```python
from build123d import *

# Parameters (mm, degrees)
CROQUIS1_W              = 21
CROQUIS1_H              = 20
SALIENTE_EXTRUIR1_DEPTH = 5
CROQUIS2_R              = 1.35
CORTAR_EXTRUIR1_DEPTH   = 6
CROQUIS3_R              = 2.5
CORTAR_EXTRUIR2_DEPTH   = 2
CROQUIS4_R              = 2.1
CORTAR_EXTRUIR3_DEPTH   = 6
CROQUIS5_R              = 3.825
CORTAR_EXTRUIR4_DEPTH   = 4
CROQUIS7_W              = 21
CROQUIS7_H              = 20
CORTAR_EXTRUIR5_DEPTH   = 2
CROQUIS8_W              = 3
CROQUIS8_H              = 20
SALIENTE_EXTRUIR2_DEPTH = 11
CROQUIS9_R              = 2.1
CORTAR_EXTRUIR6_DEPTH   = 4
CROQUIS10_R             = 3.825
CORTAR_EXTRUIR7_DEPTH   = 2
CROQUIS11_W             = 32
CROQUIS11_H             = 20
CROQUIS11_R             = 3.825
CROQUIS11_R_2           = 1.35
SALIENTE_EXTRUIR3_DEPTH = 0.5


with BuildPart() as part:
    # Croquis1 → Saliente-Extruir1 (new body)
    with BuildSketch(Plane(origin=(0, 0, 0), x_dir=(0, 0, -1), z_dir=(1, 0, 0))):
        Rectangle(CROQUIS1_W, CROQUIS1_H)
    extrude(amount=SALIENTE_EXTRUIR1_DEPTH)

    # Croquis2 → Cortar-Extruir1 (cut, through all)
    with BuildSketch(Plane(origin=(5, 0, 0), x_dir=(0, 0, -1), z_dir=(1, 0, 0))):
        with Locations((-7.5, 3.5)):
            Circle(CROQUIS2_R)
        with Locations((-7.5, -6.5)):
            Circle(CROQUIS2_R)
    extrude(amount=-CORTAR_EXTRUIR1_DEPTH, mode=Mode.SUBTRACT)

    # Croquis3 → Cortar-Extruir2 (cut)
    with BuildSketch(Plane.ZY):
        with Locations((7.5, 3.5)):
            Circle(CROQUIS3_R)
        with Locations((7.5, -6.5)):
            Circle(CROQUIS3_R)
    extrude(amount=-CORTAR_EXTRUIR2_DEPTH, mode=Mode.SUBTRACT)

    # Croquis4 → Cortar-Extruir3 (cut, through all)
    with BuildSketch(Plane(origin=(5, 0, 0), x_dir=(0, 0, -1), z_dir=(1, 0, 0))):
        with Locations((4.7, 0)):
            Circle(CROQUIS4_R)
    extrude(amount=-CORTAR_EXTRUIR3_DEPTH, mode=Mode.SUBTRACT)

    # Croquis5 → Cortar-Extruir4 (cut)
    with BuildSketch(Plane(origin=(5, 0, 0), x_dir=(0, 0, -1), z_dir=(1, 0, 0))):
        with Locations((4.7, 0)):
            Circle(CROQUIS5_R)
    extrude(amount=-CORTAR_EXTRUIR4_DEPTH, mode=Mode.SUBTRACT)

    # Croquis7 → Cortar-Extruir5 (cut)
    with BuildSketch(Plane(origin=(5, 0, 0), x_dir=(0, 0, -1), z_dir=(1, 0, 0))):
        Rectangle(CROQUIS7_W, CROQUIS7_H)
    extrude(amount=-CORTAR_EXTRUIR5_DEPTH, mode=Mode.SUBTRACT)

    # Croquis8 → Saliente-Extruir2 (add)
    with BuildSketch(Plane.XY.offset(10.5)):
        with Locations((1.5, 0)):
            Rectangle(CROQUIS8_W, CROQUIS8_H)
    extrude(amount=SALIENTE_EXTRUIR2_DEPTH)

    # Croquis9 → Cortar-Extruir6 (cut, through all)
    with BuildSketch(Plane(origin=(3, 0, 0), x_dir=(0, 0, -1), z_dir=(1, 0, 0))):
        with Locations((-16.65, 0)):
            Circle(CROQUIS9_R)
    extrude(amount=-CORTAR_EXTRUIR6_DEPTH, mode=Mode.SUBTRACT)

    # Croquis10 → Cortar-Extruir7 (cut)
    with BuildSketch(Plane(origin=(3, 0, 0), x_dir=(0, 0, -1), z_dir=(1, 0, 0))):
        with Locations((-16.65, 0)):
            Circle(CROQUIS10_R)
    extrude(amount=-CORTAR_EXTRUIR7_DEPTH, mode=Mode.SUBTRACT)

    # Croquis11 → Saliente-Extruir3 (add)
    with BuildSketch(Plane(origin=(3, 0, 0), x_dir=(0, 0, -1), z_dir=(1, 0, 0))):
        with Locations((-5.5, 0)):
            Rectangle(CROQUIS11_W, CROQUIS11_H)
        with Locations((-16.65, 0)):
            Circle(CROQUIS11_R, mode=Mode.SUBTRACT)
        with Locations((-7.5, 3.5)):
            Circle(CROQUIS11_R_2, mode=Mode.SUBTRACT)
        with Locations((-7.5, -6.5)):
            Circle(CROQUIS11_R_2, mode=Mode.SUBTRACT)
        with Locations((4.7, 0)):
            Circle(CROQUIS11_R, mode=Mode.SUBTRACT)
    extrude(amount=SALIENTE_EXTRUIR3_DEPTH)


solid = part.part
```
Work out the finished part from the listing and answer in its coordinate system (mm). A direction names the side the tool comes from. Give positions to 0.01 mm unless a question says otherwise; leave off trailing zeros. Loops run counter-clockwise (first coordinate to the right, second up) from the corner with the lowest first, then second, coordinate; pieces in that order, holes last. Notation, with made-up numbers: (52, -39.75) -> (96, -39.75) arc R10 ccw to (96, -32.75) -> close; hole circle Ø10 at (-6, 44). An arc over 180 degrees is marked (long way). Put each result on its own line as item: value. Start each with the question number.
Item 1: The part is cut by section B-B (z = 7.5). Give the vertices of the cut face in (x, y).
Item 2: The part is cut by section A-A (x = 2.65). Give the vertices of the cut face in (y, z) (3 decimals).
Item 3: Which of the six approach directions +Z, -Z, +X, -X, +Y, -Y give full straight-line access (tool end or side, diameter ignored) to faces 1 (the face through (2, 10, 6)), 2 (the face through (1, -2, 15)), 3 (the face through (0.986, 4.251, 9.885))?
Item 4: The mould has two halves that part along Y. Classify faces 4 (the face through (1, -2, -6)), 5 (the face through (2, -10, 6)), 6 (the face through (3.5, 0, 6)): released by +Y, released by -Y, zero draft, split by the parting line, or undercut.
Item 5: Find the intervals of material crossed by L1, parallel to Y at x = 2.5, z = 7.5; L2, parallel to Y at x = 3.25, z = -4.7 (3 decimals); L3, parallel to Z at x = 2.55, y = 0.25, in increasing order. Write a range as [from, to].
Item 6: Each of these flat-tipped pins is pushed along its axis until it touches: P1, Ø4, axis at y = 1.5, z = 17, coming from the +X side; P2, Ø3.5, axis at y = 3.5, z = 7.5, coming from the -X side; P3, Ø2.5, axis at y = -6.5, z = 7.5, coming from the +X side. Where does it stop, or does it pass through?
Item 7: The part is cut by section D-D (z = 16.65). Give the vertices of the cut face in (x, y) (3 decimals).
Item 8: The part is cut by section C-C (y = 0). Give the vertices of the cut face in (x, z) (3 decimals).
Answers below:
1. outline: (0, -10) -> (3.5, -10) -> (3.5, -7.85) -> (2, -7.85) -> (2, -9) -> (0, -9) -> close; (0, -4) -> (2, -4) -> (2, -5.15) -> (3.5, -5.15) -> (3.5, 2.15) -> (2, 2.15) -> (2, 1) -> (0, 1) -> close; (0, 6) -> (2, 6) -> (2, 4.85) -> (3.5, 4.85) -> (3.5, 10) -> (0, 10) -> close
2. outline: (-10, -10.5) -> (10, -10.5) -> (10, 21.5) -> (-10, 21.5) -> close; hole circle Ø2.7 at (-6.5, 7.5); hole circle Ø7.65 at (0, -4.7); hole circle Ø7.65 at (0, 16.65); hole circle Ø2.7 at (3.5, 7.5)
3. face 1: +Z, -Z, +X, -X, +Y
3. face 2: +X
3. face 3: -X
4. face 4: undercut
4. face 5: released by -Y
4. face 6: zero draft
5. L1: [-10, -7.85], [-5.15, 2.15], [4.85, 10]
5. L2: [-10, -3.825], [3.825, 10]
5. L3: [-10.5, -8.52], [-0.88, 12.83], [20.47, 21.5]
6. P1: x = 1
6. P2: x = 2
6. P3: through
7. outline: (0, -10) -> (3.5, -10) -> (3.5, -3.825) -> (1, -3.825) -> (1, -2.1) -> (0, -2.1) -> close; (0, 2.1) -> (1, 2.1) -> (1, 3.825) -> (3.5, 3.825) -> (3.5, 10) -> (0, 10) -> close
8. outline: (0, -10.5) -> (3.5, -10.5) -> (3.5, -8.525) -> (1, -8.525) -> (1, -6.8) -> (0, -6.8) -> close; (0, -2.6) -> (1, -2.6) -> (1, -0.875) -> (3.5, -0.875) -> (3.5, 12.825) -> (1, 12.825) -> (1, 14.55) -> (0, 14.55) -> close; (0, 18.75) -> (1, 18.75) -> (1, 20.475) -> (3.5, 20.475) -> (3.5, 21.5) -> (0, 21.5) -> close
